Could you check a few things on this drawing? It's one solid part, dimensions in mm from its lowest x, y, z. A direction names the side the tool comes from. Round coordinates to 2 decimals unless told otherwise and drop trailing zeros. Loops run counter-clockwise (first coordinate to the right, second up) from the corner with the lowest first, then second, coordinate; pieces in that order, holes last. Notation, with made-up numbers: M -28.75,-19.75 L 9.25,-19.75 A19 cw 9.25,10.25 Z; hole C -14,-0.75 d4. An arc over 180 degrees is marked long. Answer as a JSON object with one key per item and string values.
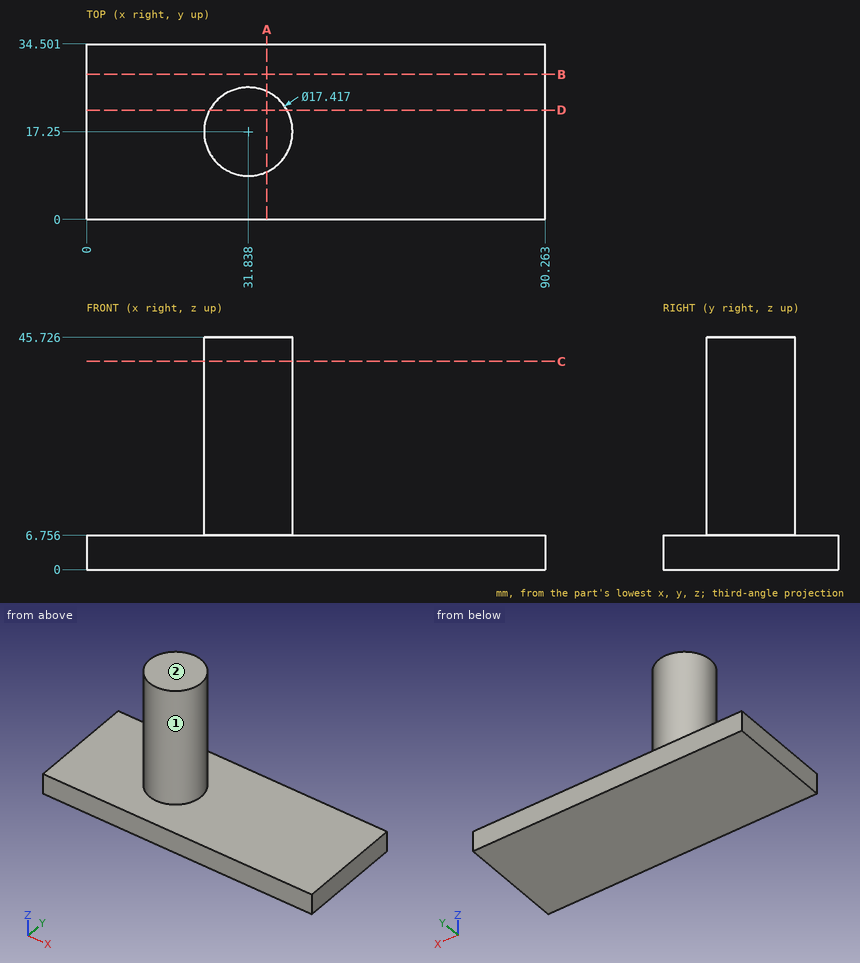
Item 1: I want a section at C-C, the plane z = 41. Please give me the cut outline in (x, y), then the cut area to 3 significant figures.
Resolved:
{"outline": "C 31.84,17.25 d17.42", "area": "238 mm²"}
Item 2: I want a section at D-D, the plane y = 21.5. Please give me the cut outline in (x, z).
Resolved:
{"outline": "M 0,0 L 90.26,0 L 90.26,6.76 L 39.44,6.76 L 39.44,45.73 L 24.24,45.73 L 24.24,6.76 L 0,6.76 Z"}
Item 3: I want a section at B-B, the plane y = 28.5. Please give me the cut outline in (x, z), then the cut area to 3 significant figures.
Resolved:
{"outline": "M 0,0 L 90.26,0 L 90.26,6.76 L 0,6.76 Z", "area": "610 mm²"}
Item 4: Please list where these lines run through material, in increasing order: probe 1 along Z at (x, y) = (48.5, 8); probe 2 along Y at (x, z) = (28, 40) (1 decimal); probe 3 along X at (y, z) = (14, 27.5). Write a range as from..to.
Resolved:
{"probe 1": "0..6.76", "probe 2": "9.4..25.1", "probe 3": "23.76..39.92"}
Item 5: On a 3-axis mill with a long thin cutter (end or side, diameter ignored), from which of +Z, -Z, +X, -X, +Y, -Y can I reach the whole of each face in a straight line? I mean the marked faces 1 and 2. Say none if no direction works.
Resolved:
{"face 1": "+Z", "face 2": "+Z, +X, -X, +Y, -Y"}
Item 6: I want a section at A-A, the plane x = 35.5. Please give me the cut outline in (y, z), then the cut area to 3 significant figures.
Resolved:
{"outline": "M 0,0 L 34.5,0 L 34.5,6.76 L 25.15,6.76 L 25.15,45.73 L 9.35,45.73 L 9.35,6.76 L 0,6.76 Z", "area": "849 mm²"}
Item 7: I'm going to push flat-ended pins straight in: pin 1 Ø10 at (y, z) = (15, 12.5) entering from -X; pin 2 Ø1 at (x, z) = (38, 15) entering from -Y (1 decimal); pin 3 Ø3 at (y, z) = (9, 33) entering from +X. Where does each tip first touch, or does it pass through?
Resolved:
{"pin 1": "x = 23.13", "pin 2": "y = 10.6", "pin 3": "x = 37.34"}
